from build123d import *

# Parameters (mm, degrees)
SKETCH_1_W       = 37.5
SKETCH_1_H       = 18.5
SKETCH_1_R       = 1.4
EXTRUDE_1_DEPTH  = 3.5
SKETCH_2_W       = 4
SKETCH_2_H       = 5.6
EXTRUDE_2_DEPTH  = 3
CHAMFER_1_SIZE   = 3.077683537
CHAMFER_1_SIZE_2 = 1


with BuildPart() as part:
    # Эскиз1 → Бобышка-Вытянуть1 (new body)
    with BuildSketch(Plane.XY):
        with Locations((18.75, -9.25)):
            Rectangle(SKETCH_1_W, SKETCH_1_H)
        with Locations((8.75, -10.7)):
            Circle(SKETCH_1_R, mode=Mode.SUBTRACT)
        with Locations((28.75, -10.7)):
            Circle(SKETCH_1_R, mode=Mode.SUBTRACT)
    extrude(amount=EXTRUDE_1_DEPTH)

    # Эскиз2 → Бобышка-Вытянуть2 (add)
    with BuildSketch(Plane.XY.offset(3.5)):
        with Locations((19, -15.2)):
            Rectangle(SKETCH_2_W, SKETCH_2_H)
        with Locations((19, -6.2)):
            Rectangle(SKETCH_2_W, SKETCH_2_H)
    extrude(amount=EXTRUDE_2_DEPTH)

    # Фаска1
    # the kernel refuses this chamfer: 3.077683537, 1 mm, written as the material it takes off along each edge
    with BuildSketch(Plane(origin=(9.012519835, -3.4, 6.5), x_dir=(0, 0.011906840413017355, -0.9999291110630687), z_dir=(1, 0, 0))) as chamfer_1_piece_1_section:
        Polygon((CHAMFER_1_SIZE * 0.99992911112, -CHAMFER_1_SIZE * 0.0119068404137), (-CHAMFER_1_SIZE_2 * 0.011906840413, -CHAMFER_1_SIZE_2 * 0.999929111063), (0, 0), align=None)
    chamfer_1_piece_1 = extrude(amount=19.97496033, mode=Mode.PRIVATE)
    chamfer_1_piece_1 = split(chamfer_1_piece_1, bisect_by=Plane(origin=(19, -3.706604024, 3.5), z_dir=(0, 0, 1)), keep=Keep.TOP, mode=Mode.PRIVATE)
    add(chamfer_1_piece_1, mode=Mode.SUBTRACT)
    with BuildSketch(Plane(origin=(21, 4.587480165, 6.5), x_dir=(0.011906840413017495, 0, -0.9999291110630687), z_dir=(0, -1, 0))) as chamfer_1_piece_2_section:
        Polygon((CHAMFER_1_SIZE * 0.99992911112, -CHAMFER_1_SIZE * 0.0119068404137), (-CHAMFER_1_SIZE_2 * 0.011906840413, -CHAMFER_1_SIZE_2 * 0.999929111063), (0, 0), align=None)
    chamfer_1_piece_2 = extrude(amount=21.57496033, mode=Mode.PRIVATE)
    chamfer_1_piece_2 = split(chamfer_1_piece_2, bisect_by=Plane(origin=(20.693395976, -6.2, 3.5), z_dir=(0, 0, 1)), keep=Keep.TOP, mode=Mode.PRIVATE)
    add(chamfer_1_piece_2, mode=Mode.SUBTRACT)
    with BuildSketch(Plane(origin=(28.987480165, -9, 6.5), x_dir=(0, -0.011906840413017495, -0.9999291110630687), z_dir=(-1, 0, 0))) as chamfer_1_piece_3_section:
        Polygon((CHAMFER_1_SIZE * 0.99992911112, -CHAMFER_1_SIZE * 0.0119068404137), (-CHAMFER_1_SIZE_2 * 0.011906840413, -CHAMFER_1_SIZE_2 * 0.999929111063), (0, 0), align=None)
    chamfer_1_piece_3 = extrude(amount=19.97496033, mode=Mode.PRIVATE)
    chamfer_1_piece_3 = split(chamfer_1_piece_3, bisect_by=Plane(origin=(19, -8.693395976, 3.5), z_dir=(0, 0, 1)), keep=Keep.TOP, mode=Mode.PRIVATE)
    add(chamfer_1_piece_3, mode=Mode.SUBTRACT)
    with BuildSketch(Plane(origin=(17, -16.987480165, 6.5), x_dir=(-0.011906840413017495, 0, -0.9999291110630687), z_dir=(0, 1, 0))) as chamfer_1_piece_4_section:
        Polygon((CHAMFER_1_SIZE * 0.99992911112, -CHAMFER_1_SIZE * 0.0119068404137), (-CHAMFER_1_SIZE_2 * 0.011906840413, -CHAMFER_1_SIZE_2 * 0.999929111063), (0, 0), align=None)
    chamfer_1_piece_4 = extrude(amount=21.57496033, mode=Mode.PRIVATE)
    chamfer_1_piece_4 = split(chamfer_1_piece_4, bisect_by=Plane(origin=(17.306604024, -6.2, 3.5), z_dir=(0, 0, 1)), keep=Keep.TOP, mode=Mode.PRIVATE)
    add(chamfer_1_piece_4, mode=Mode.SUBTRACT)
    with BuildSketch(Plane(origin=(9.012519835, -12.4, 6.5), x_dir=(0, 0.011906840413017495, -0.9999291110630687), z_dir=(1, 0, 0))) as chamfer_1_piece_5_section:
        Polygon((CHAMFER_1_SIZE * 0.99992911112, -CHAMFER_1_SIZE * 0.0119068404137), (-CHAMFER_1_SIZE_2 * 0.011906840413, -CHAMFER_1_SIZE_2 * 0.999929111063), (0, 0), align=None)
    chamfer_1_piece_5 = extrude(amount=19.97496033, mode=Mode.PRIVATE)
    chamfer_1_piece_5 = split(chamfer_1_piece_5, bisect_by=Plane(origin=(19, -12.706604024, 3.5), z_dir=(0, 0, 1)), keep=Keep.TOP, mode=Mode.PRIVATE)
    add(chamfer_1_piece_5, mode=Mode.SUBTRACT)
    with BuildSketch(Plane(origin=(21, -4.412519835, 6.5), x_dir=(0.011906840413017495, 0, -0.9999291110630687), z_dir=(0, -1, 0))) as chamfer_1_piece_6_section:
        Polygon((CHAMFER_1_SIZE * 0.99992911112, -CHAMFER_1_SIZE * 0.0119068404137), (-CHAMFER_1_SIZE_2 * 0.011906840413, -CHAMFER_1_SIZE_2 * 0.999929111063), (0, 0), align=None)
    chamfer_1_piece_6 = extrude(amount=21.57496033, mode=Mode.PRIVATE)
    chamfer_1_piece_6 = split(chamfer_1_piece_6, bisect_by=Plane(origin=(20.693395976, -15.2, 3.5), z_dir=(0, 0, 1)), keep=Keep.TOP, mode=Mode.PRIVATE)
    add(chamfer_1_piece_6, mode=Mode.SUBTRACT)
    with BuildSketch(Plane(origin=(28.987480165, -18, 6.5), x_dir=(0, -0.011906840413017495, -0.9999291110630687), z_dir=(-1, 0, 0))) as chamfer_1_piece_7_section:
        Polygon((CHAMFER_1_SIZE * 0.99992911112, -CHAMFER_1_SIZE * 0.0119068404137), (-CHAMFER_1_SIZE_2 * 0.011906840413, -CHAMFER_1_SIZE_2 * 0.999929111063), (0, 0), align=None)
    chamfer_1_piece_7 = extrude(amount=19.97496033, mode=Mode.PRIVATE)
    chamfer_1_piece_7 = split(chamfer_1_piece_7, bisect_by=Plane(origin=(19, -17.693395976, 3.5), z_dir=(0, 0, 1)), keep=Keep.TOP, mode=Mode.PRIVATE)
    add(chamfer_1_piece_7, mode=Mode.SUBTRACT)
    with BuildSketch(Plane(origin=(17, -25.987480165, 6.5), x_dir=(-0.011906840413017495, 0, -0.9999291110630687), z_dir=(0, 1, 0))) as chamfer_1_piece_8_section:
        Polygon((CHAMFER_1_SIZE * 0.99992911112, -CHAMFER_1_SIZE * 0.0119068404137), (-CHAMFER_1_SIZE_2 * 0.011906840413, -CHAMFER_1_SIZE_2 * 0.999929111063), (0, 0), align=None)
    chamfer_1_piece_8 = extrude(amount=21.57496033, mode=Mode.PRIVATE)
    chamfer_1_piece_8 = split(chamfer_1_piece_8, bisect_by=Plane(origin=(17.306604024, -15.2, 3.5), z_dir=(0, 0, 1)), keep=Keep.TOP, mode=Mode.PRIVATE)
    add(chamfer_1_piece_8, mode=Mode.SUBTRACT)


solid = part.part
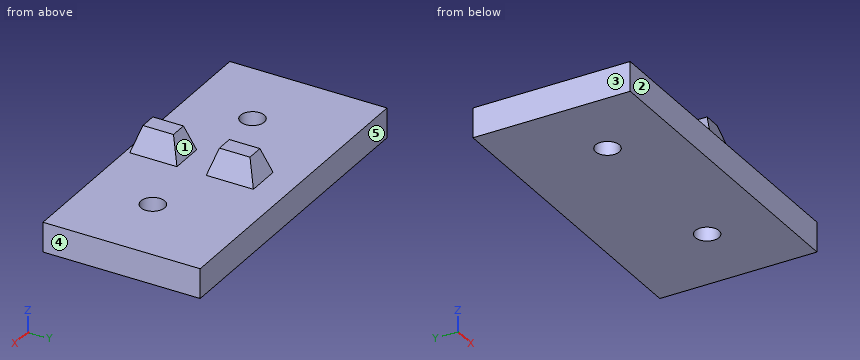
CAD build for the part. Positions are in the model's coordinates, mm. Face numbers are marked on the shaded views. A direction names the side the tool comes from. Round coordinates to 2 decimals unless told otherwise and drop trailing zeros. Write each loop counter-clockwise with the first axis right and the second up, starting at its lowest first coordinate (ties: lowest second). Pieces come first, ordered by that corner, then holes. Notation, with made-up numbers: M 2,61.25 L 38,61.25 A18 cw 38,76.25 Z; hole C 17,66 d1. An arc over 180 degrees is marked long. Use a Markdown table: item, result. Add a question column.
1. 3-axis set-ups, long thin cutter, end or side, ignore diameter. For the marked faces 1 and 2: which of +Z, -Z, +X, -X, +Y, -Y reach the whole face in a straight line?
2. Slice it at C-C on z = 5.75. Give the cut face in (x, y).
3. Pull direction X, two halves, no side cores. Call the marked faces 3, 4 and 5: released by +X, released by -X, zero draft, split by the parting line, or undercut.
4. Flat gauge pins, fed straight in: P1, Ø3, axis at y = -4, z = 4.5, coming from the -X side; P2, Ø1.7, axis at x = 28.75, y = -10.7, coming from the +Z side; P3, Ø4.5, axis at x = 8.75, y = -10.7, coming from the +Z side. Where does each tip first touch, or does it go through?
5. Slice it at A-A on y = -10.7. Give the cut face in (x, z), then the cut area to 3 significant figures.
6. Slice it at D-D on z = 2.25. Give the cut face in (x, y), then the cut area to 3 significant figures.
7. Slice it at B-B on x = 8.75. Give the cut face in (y, z), then the cut area to 4 significant figures.
8. Drill centre lines: probe 1 along Y at (x, z) = (28.75, 1.9); probe 2 along X at (y, z) = (-10.5, 0.5); probe 3 along X at (y, z) = (-9.75, 2). Where is each one in solid material? Low to high.
Reply:
| question | item | result |
|---|---|---|
| 1 | face 1 | +Z, +X, -X |
| 1 | face 2 | +Z, -Z, +X, -X, -Y |
| 2 | outline | M 17.76,-17.24 L 20.24,-17.24 L 20.24,-13.16 L 17.76,-13.16 Z; M 17.76,-8.24 L 20.24,-8.24 L 20.24,-4.16 L 17.76,-4.16 Z |
| 3 | face 3 | released by -X |
| 3 | face 4 | released by +X |
| 3 | face 5 | zero draft |
| 4 | P1 | stops at x = 0 |
| 4 | P2 | passes through |
| 4 | P3 | stops at z = 3.5 |
| 5 | outline | M 0,0 L 7.35,0 L 7.35,3.5 L 0,3.5 Z; M 10.15,0 L 27.35,0 L 27.35,3.5 L 10.15,3.5 Z; M 30.15,0 L 37.5,0 L 37.5,3.5 L 30.15,3.5 Z |
| 5 | area | 112 mm^2 |
| 6 | outline | M 0,-18.5 L 37.5,-18.5 L 37.5,0 L 0,0 Z; hole C 8.75,-10.7 d2.8; hole C 28.75,-10.7 d2.8 |
| 6 | area | 681 mm^2 |
| 7 | outline | M -18.5,0 L -12.1,0 L -12.1,3.5 L -18.5,3.5 Z; M -9.3,0 L 0,0 L 0,3.5 L -9.3,3.5 Z |
| 7 | area | 54.95 mm^2 |
| 8 | probe 1 | y = -18.5 to -12.1, -9.3 to 0 |
| 8 | probe 2 | x = 0 to 7.36, 10.14 to 27.36, 30.14 to 37.5 |
| 8 | probe 3 | x = 0 to 7.72, 9.78 to 27.72, 29.78 to 37.5 |
